Verification items for this drawing (mm, ordinates from the low corner). Give positions to 0.01 mm unless a question says otherwise; leave off trailing zeros. Order: outer loops, then holes, each group sorted by start corner. A loop starts at its lowest first (then second) coordinate and runs counter-clockwise, first axis right, second up.
(1) Mould release check, pull along X, two halves, no side actions. Record for the marked faces 1, 2 and 3: pulls with the +X half, pulls with the -X half, needs draft (parallel to the pull), parting line crosses it, or undercut.
(2) Sectioned sample at A-A on y = 5.5. Record the cut outline in (x, z), plus the area to 3 significant figures.
(3) Gauge pin test, flat end, axial feed: pin 1 (13 mm diameter, centred on x = 9.4, y = 37.49, fed in from -Z). Record the tip position at first contact, or that the pin passes through.
(4) Scan lines: L1, parallel to X at y = 63, z = 1.25 (1 decimal); L2, parallel to X at y = 63.5, z = 1.75 (1 decimal). Record each from-to range of solid material in increasing order.
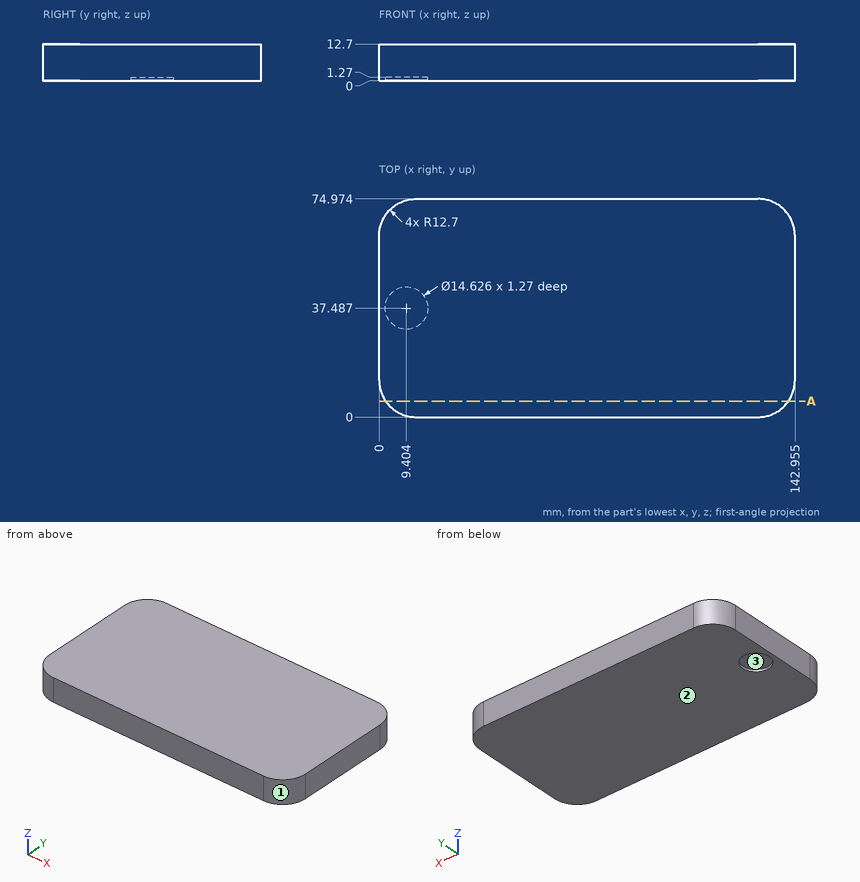
Ans:
1. face 1: pulls with the +X half
1. face 2: needs draft
1. face 3: undercut
2. outline: (2.24, 0) - (140.72, 0) - (140.72, 12.7) - (2.24, 12.7) - close
2. area: 1,760 mm2
3. pin 1: stops at z = 1.27
4. L1: x = 0 to 142.9
4. L2: x = 0.1 to 142.9
